from build123d import *

# Parameters (mm, degrees)
SKETCH_1_W          = 23
SKETCH_1_H          = 17
EXTRUDE_1_DEPTH     = 6.5
SKETCH_2_W          = 20
SKETCH_2_H          = 15.5
CUT_EXTRUDE_1_DEPTH = 5
SKETCH_3_W          = 23
SKETCH_3_H          = 1.5
EXTRUDE_2_DEPTH     = 12.6
EXTRUDE_3_DEPTH     = 3
HOLE_WIZARD_M3_1_D  = 3.2
EXTRUDE_START       = 10
EXTRUDE_6_DEPTH     = 1.5
FILLET_1_R          = 3
SKETCH_10_W         = 1.5
SKETCH_10_H         = 9
EXTRUDE_7_DEPTH     = 9.486304789
SKETCH_11_W         = 1
SKETCH_11_H         = 9
EXTRUDE_8_DEPTH     = 14
HOLE_WIZARD_M3_2_D  = 3.2
CUT_EXTRUDE_2_REACH = 31.686
SKETCH_14_W         = 6
SKETCH_14_H         = 3.5


# Read off the part's stored shape, not the designer's step: 凸台-拉伸6
with BuildPart() as part:
    # 草图1 → 凸台-拉伸1 (new body)
    with BuildSketch(Plane.XY):
        Rectangle(SKETCH_1_W, SKETCH_1_H)
    extrude(amount=EXTRUDE_1_DEPTH)

    # 草图2 → 切除-拉伸1 (cut)
    with BuildSketch(Plane.XY.offset(6.5)):
        with Locations((0, -0.75)):
            Rectangle(SKETCH_2_W, SKETCH_2_H)
    extrude(amount=-CUT_EXTRUDE_1_DEPTH, mode=Mode.SUBTRACT)

    # 草图3 → 凸台-拉伸2 (add)
    with BuildSketch(Plane(origin=(0, 0, 0), x_dir=(-1, 0, 0), z_dir=(0, 0, -1))):
        with Locations((0, -7.75)):
            Rectangle(SKETCH_3_W, SKETCH_3_H)
    extrude(amount=EXTRUDE_2_DEPTH)

    # 草图4 → 凸台-拉伸3 (add)
    with BuildSketch(Plane(origin=(0, -7, 0), x_dir=(1, 0, 0), z_dir=(0, 1, 0))):
        Polygon((5.080682369, 6.4), (2.540341184, 10.8), (-2.540341184, 10.8), (-5.080682369, 6.4), (-2.540341184, 2), (2.540341184, 2), align=None)
        Polygon((3.348631561, 6.4), (1.674315781, 9.3), (-1.674315781, 9.3), (-3.348631561, 6.4), (-1.674315781, 3.5), (1.674315781, 3.5), align=None, mode=Mode.SUBTRACT)
    extrude(amount=EXTRUDE_3_DEPTH)

    # M3 间隙孔1 (through all)
    with Locations(Plane(origin=(0, -7, 0), x_dir=(1, 0, 0), z_dir=(0, 1, 0))):
        with Locations((0, 6.4)):
            Hole(HOLE_WIZARD_M3_1_D / 2)

    # 凸台-拉伸6 outline → 凸台-拉伸6 (add)
    with BuildSketch(Plane.YZ.offset(EXTRUDE_START)):
        Polygon((-7, -10.266991259), (3.266991259, 0), (-7, 0), align=None)
    extrude(amount=EXTRUDE_6_DEPTH)

    # 圆角1
    fillet_1_edges = [part.edges().sort_by_distance(p)[0] for p in [
        (-11.5, -7.75, -12.6),
        (11.5, -7.75, -12.6),
    ]]
    fillet(fillet_1_edges, radius=FILLET_1_R)

    # 草图10 → 凸台-拉伸7 (add)
    with BuildSketch(Plane(origin=(0, 0, 0), x_dir=(-1, 0, 0), z_dir=(0, 0, -1))):
        with Locations((10.75, 2.3)):
            Rectangle(SKETCH_10_W, SKETCH_10_H)
    extrude(amount=EXTRUDE_7_DEPTH)

    # 草图11 → 凸台-拉伸8 (add)
    with BuildSketch(Plane.ZY.offset(11.5)):
        with Locations((-8.986304789, 2.3)):
            Rectangle(SKETCH_11_W, SKETCH_11_H)
    extrude(amount=EXTRUDE_8_DEPTH)

    # M3 间隙孔2 (through all)
    with Locations(Plane.XY.offset(-8.486304789)):
        with Locations((-18.5, 2.3)):
            Hole(HOLE_WIZARD_M3_2_D / 2)

    # 草图14 → 切除-拉伸2 (cut, up to next)
    with BuildSketch(Plane(origin=(0, 0, 0), x_dir=(-1, 0, 0), z_dir=(0, 0, -1)), mode=Mode.PRIVATE) as cut_extrude_2_sk1:
        with Locations((0, -2.75)):
            Rectangle(SKETCH_14_W, SKETCH_14_H)
    cut_extrude_2_tool1 = extrude(cut_extrude_2_sk1.sketch, amount=-CUT_EXTRUDE_2_REACH, mode=Mode.PRIVATE) & part.part
    add(cut_extrude_2_tool1.solids().sort_by_distance((0, -2.75, 0))[0], mode=Mode.SUBTRACT)


solid = part.part
The listing builds one solid part. Answer for the finished solid, in the listing's coordinates (mm). A direction names the side the tool comes from. Coordinates: 2 decimals unless noted, no trailing zeros. Order: outer loops, then holes, each group sorted by start corner. A loop starts at its lowest first (then second) coordinate and runs counter-clockwise, first axis right, second up. Notation, with made-up numbers: M -26,15.25 L -10,15.25 A11 cw -10,27.25 Z; hole C 60.5,-28 d6. An arc over 180 degrees is marked long. Use CSV: the item, a comma, the result in double quotes.
Q1. Section C-C (x = 7.5) is taken. Determine the outline of the cut face in (y, z).
Here are the results:
outline,"M -8.5,-12.6 L -7,-12.6 L -7,0 L 8.5,0 L 8.5,6.5 L 7,6.5 L 7,1.5 L -8.5,1.5 Z"
Q2. Section B-B (z = 0.75) is taken. Determine the outline of the cut face in (x, y).
Here are the results:
outline,"M -11.5,-8.5 L 11.5,-8.5 L 11.5,8.5 L -11.5,8.5 Z; hole M -3,-4.5 L 3,-4.5 L 3,-1 L -3,-1 Z"
Q3. A tool of negligible diameter and unlimited length cuts with its end or side. For faces 1 (the flat face through (3.793, -5.521, -4.169)), 2 (the flat face through (-16, 2, -9.486)), 3 (the flat face through (0, -4.5, 1)), from which of +Z, -Z, +X, -X, +Y, -Y can it reach the whole face along a straight path? Write none if from no direction.
Here are the results:
face 1,"+Y"
face 2,"-Z, +X, -X, +Y"
face 3,"+Z"
Q4. Given pin 1 Ø3 at (x, z) = (0, -7.5) entering from +Y; pin 2 Ø1.5 at (y, z) = (3, 4.5) entering from -X; pin 3 Ø10 at (x, y) = (-18.5, 2.5) entering from +Z; pin 4 Ø4 at (x, z) = (0, -6.4) entering from -Y, each flat-ended and moving along its own axis, determine where each tip first touches the part or whether it passes through.
Here are the results:
pin 1,"y = -7"
pin 2,"x = -11.5"
pin 3,"z = -8.49"
pin 4,"y = -8.5"
Q5. Determine the mould class of faces 4 (the flat face through (-0.1, -0.6, 1.5)), 5 (the flat face through (0, -1, 1)), 6 (the flat face through (-17, 1, -8.486)), 7 (the flat face through (-3.83, -5.52, -4.23)) for opening direction X: pulls with the +X half, pulls with the -X half, needs draft (parallel to the pull), parting line crosses it, or undercut.
Here are the results:
face 4,"undercut"
face 5,"undercut"
face 6,"needs draft"
face 7,"pulls with the -X half"
Q6. Straight lines are drawn through the part: L1, parallel to Z at x = 0, y = -8.1; L2, parallel to Y at x = -18.5, z = -9.1; L3, parallel to Y at x = -1, z = 0.25. For each, find the intervals that lie inside material, in ascending order.
Here are the results:
L1,"-12.6 to -8, -4.8 to 1.5"
L2,"-2.2 to 0.7, 3.9 to 6.8"
L3,"-8.5 to -4.5, -1 to 8.5"
Q7. Section D-D (x = 0) is taken. Determine the outline of the cut face in (y, z), then the cut area to 4 significant figures.
Here are the results:
outline,"M -8.5,-12.6 L -7,-12.6 L -7,-10.8 L -4,-10.8 L -4,-9.3 L -7,-9.3 L -7,-8 L -8.5,-8 Z; M -8.5,-4.8 L -7,-4.8 L -7,-3.5 L -4,-3.5 L -4,-2 L -7,-2 L -7,0 L -4.5,0 L -4.5,1.5 L -8.5,1.5 Z; M -1,0 L 8.5,0 L 8.5,6.5 L 7,6.5 L 7,1.5 L -1,1.5 Z"
area,"50.85 mm2"
Q8. Section A-A (x = -18.5) is taken. Determine the outline of the cut face in (y, z).
Here are the results:
outline,"M -2.2,-9.49 L 0.7,-9.49 L 0.7,-8.49 L -2.2,-8.49 Z; M 3.9,-9.49 L 6.8,-9.49 L 6.8,-8.49 L 3.9,-8.49 Z"
